Here's the drawing with two shaded views (mm, measured from the low corner). I have some questions. A direction names the side the tool comes from. Round coordinates to 2 decimals unless told otherwise and drop trailing zeros. Loops run counter-clockwise (first coordinate to the right, second up) from the corner with the lowest first, then second, coordinate; pieces in that order, holes last.
(1) Thinking about a two-plate mould opening in Z: for the marked faces 1, 2 and 3, which applies, released by +Z, released by -Z, zero draft, split by the parting line, or undercut?
(2) Which directions (+Z, -Z, +X, -X, +Y, -Y) give clear straight access to the entire face, cutting with the end or side of a thin tool? Please do the marked faces 4 and 5.
(3) I want a section at B-B on x = 9.5. Write out the boundary of the cut face in (y, z).
(4) If I drill on line 1 along Z through (x, y) = (9.5, 17); line 2 along Z through (x, y) = (9.5, 5.5); line 3 along Y through (x, z) = (7, 7), over which ranges is the centre line in solid material (lowest first)?
(5) I want a section at C-C on y = 10.5. Write out the boundary of the cut face in (x, z).
(6) I want a section at D-D on y = 17.25. Write out the boundary of the cut face in (x, z).
(7) Will these pins go through, and if not, where does the flat tip stop? pin 1 Ø5 at (y, z) = (4.5, 17) entering from +X; pin 2 Ø2 at (x, y) = (5, 10.5) entering from -Z; pin 3 Ø1.5 at (x, y) = (16.5, 17) entering from -Z.
(8) I want a section at A-A on z = 9.5. Write out the boundary of the cut face in (x, y).
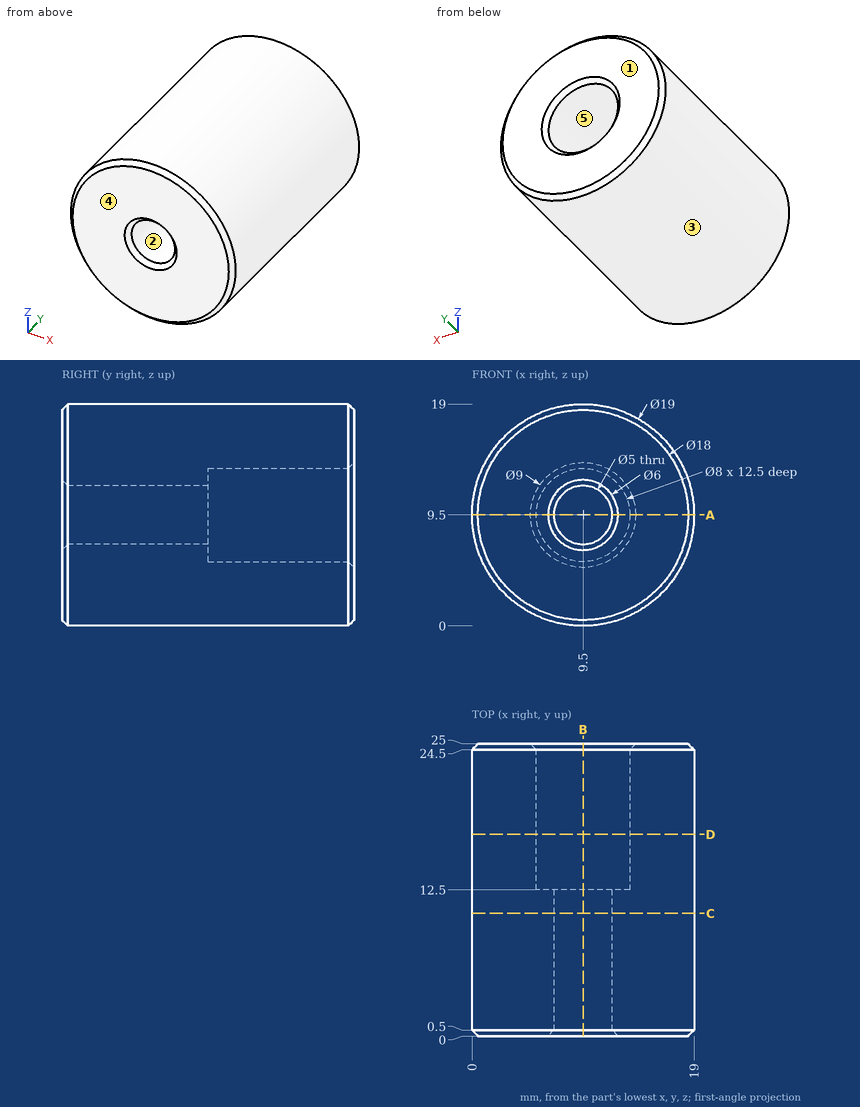
Filled sheet:
1. face 1: zero draft
1. face 2: undercut
1. face 3: split by the parting line
2. face 4: +Z, -Z, +X, -X, -Y
2. face 5: +Y
3. outline: (0, 0.5) - (0.5, 0) - (24.5, 0) - (25, 0.5) - (25, 5) - (24.5, 5.5) - (12.5, 5.5) - (12.5, 7) - (0.5, 7) - (0, 6.5) - close; (0, 12.5) - (0.5, 12) - (12.5, 12) - (12.5, 13.5) - (24.5, 13.5) - (25, 14) - (25, 18.5) - (24.5, 19) - (0.5, 19) - (0, 18.5) - close
4. line 1: z = 0 to 5.5, 13.5 to 19
4. line 2: z = 0 to 7, 12 to 19
4. line 3: y = 0 to 12.5
5. outline: circle Ø19 at (9.5, 9.5); hole circle Ø5 at (9.5, 9.5)
6. outline: circle Ø19 at (9.5, 9.5); hole circle Ø8 at (9.5, 9.5)
7. pin 1: stops at x = 17.58
7. pin 2: stops at z = 0.67
7. pin 3: stops at z = 2.35
8. outline: (0, 0.5) - (0.5, 0) - (6.5, 0) - (7, 0.5) - (7, 12.5) - (5.5, 12.5) - (5.5, 24.5) - (5, 25) - (0.5, 25) - (0, 24.5) - close; (12, 0.5) - (12.5, 0) - (18.5, 0) - (19, 0.5) - (19, 24.5) - (18.5, 25) - (14, 25) - (13.5, 24.5) - (13.5, 12.5) - (12, 12.5) - close
